The model under review builds one solid part; all positions refer to its coordinate system, in mm. Face numbers are marked on the shaded views. A direction names the side the tool comes from. Round coordinates to 2 decimals unless told otherwise and drop trailing zeros. Order: outer loops, then holes, each group sorted by start corner. A loop starts at its lowest first (then second) coordinate and runs counter-clockwise, first axis right, second up.
```python
from build123d import *

# Parameters (mm, degrees)
F1_DEPTH = 380
F2_R     = 25
F3_DEPTH = 10
F4_R     = 12.5
F5_DEPTH = 10


with BuildPart() as f1:
    # F0 (on Front) → F1 (new body)
    with BuildSketch(Plane.XZ):
        with BuildLine():
            Line((-410, -220), (410, -220))
            ThreePointArc((410, -220), (445.355339, -205.355339), (460, -170))
            Line((460, -170), (460, 170))
            ThreePointArc((460, 170), (445.355339, 205.355339), (410, 220))
            Line((410, 220), (-410, 220))
            ThreePointArc((-410, 220), (-445.355339, 205.355339), (-460, 170))
            Line((-460, 170), (-460, -170))
            ThreePointArc((-460, -170), (-445.355339, -205.355339), (-410, -220))
        make_face()
        with BuildLine():
            ThreePointArc((435, -170), (427.67767, -187.67767), (410, -195))
            Line((410, -195), (-410, -195))
            ThreePointArc((-410, -195), (-427.67767, -187.67767), (-435, -170))
            Line((-435, -170), (-435, 170))
            ThreePointArc((-435, 170), (-427.67767, 187.67767), (-410, 195))
            Line((-410, 195), (410, 195))
            ThreePointArc((410, 195), (427.67767, 187.67767), (435, 170))
            Line((435, 170), (435, -170))
        make_face(mode=Mode.SUBTRACT)
    extrude(amount=F1_DEPTH)

    # F2 (on face) → F3 (cut)
    with BuildSketch(Plane(origin=(0, 0, -220), x_dir=(1, 0, 0), z_dir=(0, 0, -1))):
        with Locations((-360, 50)):
            Circle(F2_R)
        with Locations((-360, 330)):
            Circle(F2_R)
        with Locations((360, 330)):
            Circle(F2_R)
        with Locations((360, 50)):
            Circle(F2_R)
    extrude(amount=-F3_DEPTH, mode=Mode.SUBTRACT)

    # F4 (on face) → F5 (cut)
    with BuildSketch(Plane.XY.offset(220)):
        with Locations((-360, -50)):
            Circle(F4_R)
        with Locations((-360, -330)):
            Circle(F4_R)
        with Locations((-120, -330)):
            Circle(F4_R)
        with Locations((-120, -50)):
            Circle(F4_R)
        with Locations((120, -330)):
            Circle(F4_R)
        with Locations((120, -50)):
            Circle(F4_R)
        with Locations((360, -330)):
            Circle(F4_R)
        with Locations((360, -50)):
            Circle(F4_R)
    extrude(amount=-F5_DEPTH, mode=Mode.SUBTRACT)


solid = f1.part
```
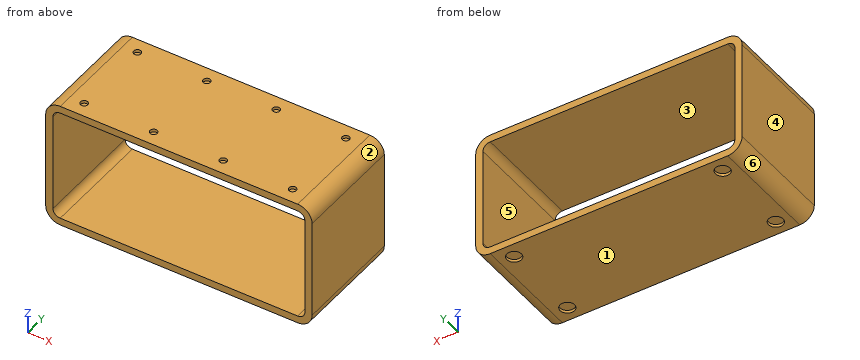
(1) Insertion check: pin 1 (7.5 mm diameter, centred on x = 120, y = -335.5, fed in from +Z); pin 2 (1.5 mm diameter, centred on y = -85.5, z = 171.5, fed in from +X). Each pin has a flat end and moves straight along its axis. Give the tip position at first contact, or say it passes through.
Data:
pin 1: stops at z = 210
pin 2: stops at x = 459.99
(2) Consider section A-A (x = 360). Write out the cut boundary in (y, z).
Data:
outline: (-380, -220) - (-355, -220) - (-355, -210) - (-305, -210) - (-305, -220) - (-75, -220) - (-75, -210) - (-25, -210) - (-25, -220) - (0, -220) - (0, -195) - (-380, -195) - close; (-380, 195) - (0, 195) - (0, 220) - (-37.5, 220) - (-37.5, 210) - (-62.5, 210) - (-62.5, 220) - (-317.5, 220) - (-317.5, 210) - (-342.5, 210) - (-342.5, 220) - (-380, 220) - close
(3) For the marked faces 5 and 6, list the 3-axis set-ups (+Z, -Z, +X, -X, +Y, -Y) from which the entire face can be reached by the end or side of a thin tool; tool diameter is ignored.
Data:
face 5: +Y, -Y
face 6: -Z, -X, +Y, -Y
(4) Consider section C-C (y = -176.5). Write out the cut boundary in (x, z), and give its area (3 significant figures).
Data:
outline: (-460, -170) arc R50 ccw to (-410, -220) - (410, -220) arc R50 ccw to (460, -170) - (460, 170) arc R50 ccw to (410, 220) - (-410, 220) arc R50 ccw to (-460, 170) - close; hole (-435, -170) arc R25 ccw to (-410, -195) - (410, -195) arc R25 ccw to (435, -170) - (435, 170) arc R25 ccw to (410, 195) - (-410, 195) arc R25 ccw to (-435, 170) - close
area: 63,900 mm2
(5) To check wall thickness, follow probe 1 along Y at (x, z) = (120, 215.75); probe 2 along Z at (x, y) = (202, -184); probe 3 along X at (y, z) = (-200.5, -4.5). State the ranges of each line that lie inside material, in increasing order.
Data:
probe 1: y = -380 to -342.5, -317.5 to -62.5, -37.5 to 0
probe 2: z = -220 to -195, 195 to 220
probe 3: x = -460 to -435, 435 to 460
(6) Consider section D-D (x = -120). Write out the cut boundary in (y, z).
Data:
outline: (-380, -220) - (0, -220) - (0, -195) - (-380, -195) - close; (-380, 195) - (0, 195) - (0, 220) - (-37.5, 220) - (-37.5, 210) - (-62.5, 210) - (-62.5, 220) - (-317.5, 220) - (-317.5, 210) - (-342.5, 210) - (-342.5, 220) - (-380, 220) - close
(7) Draft analysis for pull direction Z (two halves, no side actions). For the marked faces 1, 2, 3 and 4, state which applies: pulls with the +Z half, pulls with the -Z half, needs draft (parallel to the pull), parting line crosses it, or undercut.
Data:
face 1: pulls with the -Z half
face 2: pulls with the +Z half
face 3: undercut
face 4: needs draft
(8) Consider section B-B (z = 50). Write out the cut boundary in (x, y), and give its area (3 significant figures).
Data:
outline: (-460, -380) - (-435, -380) - (-435, 0) - (-460, 0) - close; (435, -380) - (460, -380) - (460, 0) - (435, 0) - close
area: 19,000 mm2
